from build123d import *

# Parameters (mm, degrees)
SKETCH1_W           = 762
SKETCH1_H           = 1524
SKETCH1_R           = 50.8
BOSS_EXTRUDE1_DEPTH = 6.35
SKETCH3_R           = 6.35
BOSS_EXTRUDE2_DEPTH = 9.525
LPATTERN1_COUNT     = 29
LPATTERN1_PITCH     = 25.4


with BuildPart() as part:
    # Sketch1 → Boss-Extrude1 (new body)
    with BuildSketch(Plane.XY):
        with Locations((381, 762)):
            Rectangle(SKETCH1_W, SKETCH1_H)
        with Locations((473.040992839, 1256.517236174)):
            Circle(SKETCH1_R, mode=Mode.SUBTRACT)
        with Locations((195.985521076, 818.027867477)):
            Circle(SKETCH1_R, mode=Mode.SUBTRACT)
        with Locations((573.391793635, 338.089254973)):
            Circle(SKETCH1_R, mode=Mode.SUBTRACT)
    extrude(amount=BOSS_EXTRUDE1_DEPTH)

    # Sketch3 → Boss-Extrude2 (add, symmetric)
    with BuildSketch(Plane.XY.offset(3.175)):
        with Locations(Location((25.4, 1498.6, 0), (0, 0, 180))):
            Circle(SKETCH3_R)
    boss_extrude2 = extrude(amount=BOSS_EXTRUDE2_DEPTH, both=True)

    # LPattern1: Boss-Extrude2 ×29
    with Locations(*[(i * LPATTERN1_PITCH, 0, 0) for i in range(1, LPATTERN1_COUNT)]):
        add(boss_extrude2)


solid = part.part
Input: part model. Units: mm. Frame: model coordinates. Round coordinates to 2 decimals unless told otherwise and drop trailing zeros. Order: outer loops, then holes, each group sorted by start corner. A loop starts at its lowest first (then second) coordinate and runs counter-clockwise, first axis right, second up. Notation, with made-up numbers: (5, 83) - (23, 83) arc R25 ccw to (23, 109) - close; hole circle Ø3 at (15, 70). An arc over 180 degrees is marked (long way). Answer as a JSON object with one key per item and string values. Group by question number.
(1) Pin query (flat end, axial travel): P1, Ø1.5, axis at y = 342, z = 6, coming from the -X side; P2, Ø2, axis at x = 194, y = 939, coming from the +Z side; P3, Ø1, axis at x = 580, y = 448.5, coming from the -Z side; P4, Ø5, axis at y = 367, z = 9.5, coming from the -X side. Return the tip coordinate at first contact, or that it passes through.
(2) Cut plane B-B (y = 1129). Return loops of the section in (x, z), then the cut area to 3 significant figures.
(3) Draft query along Y for faces 1 (the face through (376, 773, 0)), 2 (the face through (435.6, 1290.85, 3.13)). Return one class per face: released by +Y, released by -Y, zero draft, split by the parting line, or undercut.
(4) Material intervals for probe 1 along Z at (x, y) = (155, 912); probe 2 along Y at (x, z) = (541, 2.5); probe 3 along Y at (x, z) = (564, 2), sorted ascending. Write a range as from..to.
(5) Cut plane A-A (z = 3). Return loops of the section in (x, y).
Here are the results:
{
 "1": {"P1": "stops at x = 0", "P2": "stops at z = 6.35", "P3": "stops at z = 0", "P4": "passes through"},
 "2": {"outline": "(0, 0) - (762, 0) - (762, 6.35) - (0, 6.35) - close", "area": "4,840 mm^2"},
 "3": {"face 1": "zero draft", "face 2": "undercut"},
 "4": {"probe 1": "z = 0..6.35", "probe 2": "y = 0..298.96, 377.22..1524", "probe 3": "y = 0..288.16, 388.01..1524"},
 "5": {"outline": "(0, 0) - (762, 0) - (762, 1524) - (0, 1524) - close; hole circle Ø101.6 at (195.99, 818.03); hole circle Ø101.6 at (473.04, 1256.52); hole circle Ø101.6 at (573.39, 338.09)"}
}
